Verification items for the finished model (mm, model axes). Face numbers are marked on the shaded views. A direction names the side the tool comes from. Give positions to 0.01 mm unless a question says otherwise; leave off trailing zeros. Loops run counter-clockwise (first coordinate to the right, second up) from the corner with the lowest first, then second, coordinate; pieces in that order, holes last. Notation, with made-up numbers: (-20, 85) - (20, 85) arc R10 cw to (20, 104) - close; hole circle Ø6 at (26.25, 89). An arc over 180 degrees is marked (long way). One line per question, with ' | ' between items. Start each with the question number.
1. Section check D-D, the plane x = -1.5. Enter the section's corners in (y, z) (3 decimals), then the cut area to 3 significant figures.
2. Tool access check on the marked faces 4, 5 and 6. Record the directions out of +Z, -Z, +X, -X, +Y, -Y that give a thin tool (end or side, any length) a straight path to the whole face; none if there is none.
3. Section check C-C, the plane z = 4. Enter the section's corners in (x, y) (3 decimals).
4. Mould release check, pull along Y, two halves, no side actions. Record for the marked faces 1, 2 and 3: +Y half, -Y half, draft (parallel to the pull), parting line (faces both ways), or undercut.
5. Depth check by flat-ended pin: pin 1 Ø4 at (x, y) = (4, -3) entering from -Z; pin 2 Ø6 at (x, y) = (-3.5, 1) entering from +Z; pin 3 Ø1.2 at (x, z) = (1, 3.5) entering from +Y (3 decimals); pin 4 Ø1.5 at (x, z) = (-3.5, 2) entering from -Y. Enter the tip coordinate at first touch or a pass-through.
6. Thickness scan on line 1 along Z through (x, y) = (2.5, -3.75); line 2 along X through (y, z) = (-1.5, 6.75); line 3 along Y through (x, z) = (1.75, 7.5) (3 decimals). Record the ranges inside material, lowest first. Write a range as from..to.
7. Section check B-B, the plane y = 5.25. Enter the section's corners in (x, z).
from build123d import *

# Parameters (mm, degrees)
SKETCH_W            = 12
SKETCH_H            = 12
PAD_DEPTH           = 1.5
SKETCH001_W         = 2.3
SKETCH001_H         = 3.35
PAD001_DEPTH        = 7
SKETCH002_W         = 11
SKETCH002_H         = 0.5
PAD002_DEPTH        = 0.25
LINEARPATTERN_COUNT = 5
LINEARPATTERN_PITCH = 2.375
SKETCH003_W         = 11
SKETCH003_H         = 1
PAD003_DEPTH        = 0.75
CHAMFER_SIZE        = 0.25
CHAMFER001_SIZE     = 0.25
CHAMFER002_SIZE     = 0.25


with BuildPart() as part:
    # Sketch → Pad (new body)
    with BuildSketch(Plane.XY):
        Rectangle(SKETCH_W, SKETCH_H)
    extrude(amount=PAD_DEPTH)

    # Sketch001 → Pad001 (join)
    with BuildSketch(Plane.XY.offset(1.5)):
        with Locations((0.85, 0)):
            Rectangle(SKETCH001_W, SKETCH001_H)
    extrude(amount=PAD001_DEPTH)

    # Sketch002 (on DatumPlane) → Pad002 (join)
    with BuildSketch(Plane(origin=(0, 0, 0), x_dir=(1, 0, 0), z_dir=(0, 0, -1))):
        with Locations((0, 4.75)):
            Rectangle(SKETCH002_W, SKETCH002_H)
    pad002 = extrude(amount=PAD002_DEPTH)

    # LinearPattern: Pad002 ×5
    with Locations(*[(0, i * LINEARPATTERN_PITCH, 0) for i in range(1, LINEARPATTERN_COUNT)]):
        add(pad002)

    # Sketch003 (on DatumPlane) → Pad003 (join)
    with BuildSketch(Plane(origin=(0, 0, 0), x_dir=(1, 0, 0), z_dir=(0, 0, -1))):
        Rectangle(SKETCH003_W, SKETCH003_H)
    extrude(amount=PAD003_DEPTH)

    # Chamfer
    chamfer_edges = [part.edges().sort_by_distance(p)[0] for p in [
        (5.5, 0, -0.75),
        (0, 0.5, -0.75),
        (0, -0.5, -0.75),
        (-5.5, 0, -0.75),
    ]]
    chamfer(chamfer_edges, length=CHAMFER_SIZE)

    # Chamfer001
    chamfer001_edges = [part.edges().sort_by_distance(p)[0] for p in [
        (6, -6, 0.75),
        (-6, -6, 0.75),
        (-6, 6, 0.75),
        (6, 6, 0.75),
    ]]
    chamfer(chamfer001_edges, length=CHAMFER001_SIZE)

    # Chamfer002
    chamfer002_edges = [part.edges().sort_by_distance(p)[0] for p in [
        (0, -6, 0),
        (6, 0, 0),
        (5.875, -5.875, 0),
        (-5.875, -5.875, 0),
        (-6, 0, 0),
        (0, 6, 0),
        (-5.875, 5.875, 0),
        (5.875, 5.875, 0),
    ]]
    chamfer(chamfer002_edges, length=CHAMFER002_SIZE)


solid = part.part
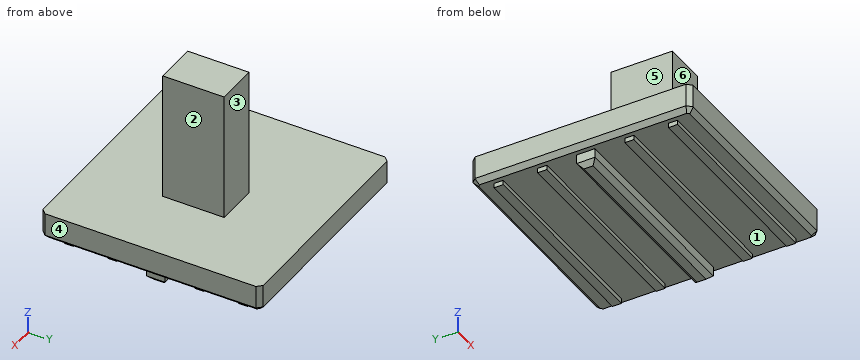
Results list:
1) outline: (-6, 0.25) - (-5.75, 0) - (-5, 0) - (-5, -0.25) - (-4.5, -0.25) - (-4.5, 0) - (-2.625, 0) - (-2.625, -0.25) - (-2.125, -0.25) - (-2.125, 0) - (-0.5, 0) - (-0.5, -0.5) - (-0.25, -0.75) - (0.25, -0.75) - (0.5, -0.5) - (0.5, 0) - (2.125, 0) - (2.125, -0.25) - (2.625, -0.25) - (2.625, 0) - (4.5, 0) - (4.5, -0.25) - (5, -0.25) - (5, 0) - (5.75, 0) - (6, 0.25) - (6, 1.5) - (-6, 1.5) - close | area: 19.1 mm²
2) face 4: +Z, -Z, +X, +Y, -Y | face 5: +Z, -X, +Y, -Y | face 6: +Z, +X, -X, -Y
3) outline: (-0.3, -1.675) - (2, -1.675) - (2, 1.675) - (-0.3, 1.675) - close
4) face 1: undercut | face 2: draft | face 3: +Y half
5) pin 1: z = -0.25 | pin 2: z = 1.5 | pin 3: y = 1.675 | pin 4: y = -6
6) line 1: 0..1.5 | line 2: -0.3..2 | line 3: -1.675..1.675
7) outline: (-6, 0.25) - (-5.75, 0) - (5.75, 0) - (6, 0.25) - (6, 1.5) - (-6, 1.5) - close
